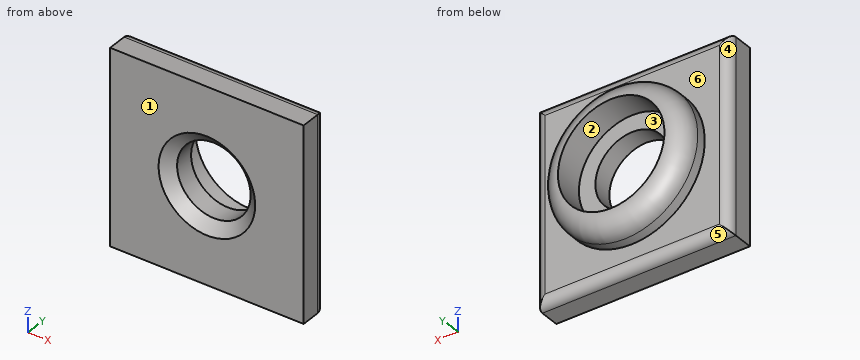
from build123d import *

# Parameters (mm, degrees)
SKETCH1_W           = 20
SKETCH1_H           = 20
SKETCH1_R           = 3.8
BOSS_EXTRUDE1_DEPTH = 3
FILLET1_R           = 1
CHAMFER1_SIZE       = 1
CHAMFER1_SIZE2      = 1.191753593
SKETCH2_R           = 7.5
SKETCH2_R_2         = 5.5
BOSS_EXTRUDE2_DEPTH = 3
FILLET2_R           = 2


with BuildPart() as part:
    # Sketch1 → Boss-Extrude1 (new body)
    with BuildSketch(Plane(origin=(0, 0, 0), x_dir=(1, 0, 0), z_dir=(0, 1, 0))):
        Rectangle(SKETCH1_W, SKETCH1_H)
        with Locations(Location((0, 0, 0), (0, 0, 270))):
            Circle(SKETCH1_R, mode=Mode.SUBTRACT)
    extrude(amount=BOSS_EXTRUDE1_DEPTH)

    # Fillet1
    fillet1_edges = [part.edges().sort_by_distance(p)[0] for p in [
        (10, 3, 0),
        (0, 3, -10),
        (-10, 3, 0),
        (0, 3, 10),
    ]]
    fillet(fillet1_edges, radius=FILLET1_R)

    # Chamfer1
    chamfer1_edges = [part.edges().sort_by_distance(p)[0] for p in [
        (0, 0, -3.8),
    ]]
    chamfer1_side = [part.faces().sort_by_distance(p)[0] for p in [
        (0, 1.5, -3.8),
    ]]
    chamfer(chamfer1_edges, length=CHAMFER1_SIZE, length2=CHAMFER1_SIZE2, reference=chamfer1_side[0])

    # Sketch2 → Boss-Extrude2 (add)
    with BuildSketch(Plane(origin=(0, 3, 0), x_dir=(1, 0, 0), z_dir=(0, 1, 0))):
        with Locations(Location((0, 0, 0), (0, 0, 270))):
            Circle(SKETCH2_R)
        with Locations(Location((0, 0, 0), (0, 0, 270))):
            Circle(SKETCH2_R_2, mode=Mode.SUBTRACT)
    extrude(amount=BOSS_EXTRUDE2_DEPTH)

    # Fillet2
    fillet2_edges = [part.edges().sort_by_distance(p)[0] for p in [
        (0, 6, -7.5),
    ]]
    fillet(fillet2_edges, radius=FILLET2_R - 0.0001)  # a hair under: the kernel refuses the full size


solid = part.part
Check sheet for the modelled part. Datum: model origin and axes. Units: mm. Face numbers are marked on the shaded views. A direction names the side the tool comes from. Round coordinates to 2 decimals unless told otherwise and drop trailing zeros. Order: outer loops, then holes, each group sorted by start corner. A loop starts at its lowest first (then second) coordinate and runs counter-clockwise, first axis right, second up. Notation, with made-up numbers: M -21,24 L 38,24 A30 ccw 38,60 Z; hole C -1.75,-32.5 d4. An arc over 180 degrees is marked long. One line per item, written item: value. Start each with the question number.
1. Section check C-C on y = 1.45. Enter the section's corners in (x, z).
2. Gauge pin test, flat ends, axial feed: P1, Ø3.5, axis at x = -1.5, z = -2.5, coming from the +Y side; P2, Ø3, axis at y = 5, z = 3.5, coming from the +X side. Record the tip position at first contact, or that the pin passes through.
3. Access from +Z, -Z, +X, -X, +Y, -Y to the whole of each face (thin tool, end or side, straight path). Record for the marked faces 5 and 6.
4. Scan lines: line 1 along X through (y, z) = (3.9, 0); line 2 along X through (y, z) = (2, 0); line 3 along Y through (x, z) = (-4.5, -3). Record each from-to range of solid material in increasing order.
5. Release check for a two-part mould opening along X. For the marked faces 1, 2, 3 and 4 record: released by +X, released by -X, zero draft, split by the parting line, or undercut.
6. Section check D-D on y = 2.7. Enter the section's corners in (x, z).
Results found:
1. outline: M -10,-10 L 10,-10 L 10,10 L -10,10 Z; hole C 0,0 d7.6
2. P1: y = 3
2. P2: x = 7.15
3. face 5: -Z, +X, -X, +Y
3. face 6: +Y
4. line 1: -7.5 to -5.5, 5.5 to 7.5
4. line 2: -10 to -3.8, 3.8 to 10
4. line 3: 0 to 3
5. face 1: zero draft
5. face 2: undercut
5. face 3: undercut
5. face 4: released by -X
6. outline: M -9.71,-9.71 L 9.71,-9.71 L 9.71,9.71 L -9.71,9.71 Z; hole C 0,0 d7.6
